Geometry: final body of the model. Coordinates: model frame, mm. Coordinates: 2 decimals unless noted, no trailing zeros. Write each loop counter-clockwise with the first axis right and the second up, starting at its lowest first coordinate (ties: lowest second). Pieces come first, ordered by that corner, then holes.
from build123d import *

# Parameters (mm, degrees)
F0_W     = 20
F0_H     = 20
F1_DEPTH = 20
F4_DEPTH = 15


with BuildPart() as f1:
    # F0 (on Top) → F1 (new body)
    with BuildSketch(Plane.XY):
        Rectangle(F0_W, F0_H)
    extrude(amount=F1_DEPTH)

    # F3 (on 3pt) → F4 (cut, symmetric)
    with BuildSketch(Plane(origin=(0, 0, 0), x_dir=(-0.7071067812, 0.7071067812, 0), z_dir=(0.7071067812, 0.7071067812, 0))):
        Polygon((14.1421356237, 0), (14.1421356237, 20), (0, 20), align=None)
    extrude(amount=F4_DEPTH, both=True, mode=Mode.SUBTRACT)


solid = f1.part
Item 1: Section B-B, the plane x = -3. Output: boundary loops of the cut face in (y, z), plus the area to 4 significant figures.
Derived:
outline: (-10, 0) - (10, 0) - (10, 7) - (-3, 20) - (-10, 20) - close
area: 315.5 mm2
Item 2: Pin query (flat end, axial travel): pin 1 (4 mm diameter, centred on x = -6, z = 5.5, fed in from +Y); pin 2 (12 mm diameter, centred on x = -6, z = 15, fed in from +Y). Return the tip coordinate at first contact, or that it passes through.
Derived:
pin 1: stops at y = 10
pin 2: stops at y = 7.49
Item 3: Section A-A, the plane z = 9.25. Output: boundary loops of the cut face in (x, y), plus the area to 3 significant figures.
Derived:
outline: (-10, -10) - (10, -10) - (10, 10) - (-0.75, 10) - (-10, 0.75) - close
area: 357 mm2
Item 4: Material intervals for probe 1 along Y at (x, z) = (-4.25, 16.75); probe 2 along X at (y, z) = (4.25, 10.5); probe 3 along Z at (x, y) = (-3, 8.25), sorted ascending.
Derived:
probe 1: y = -10 to -1
probe 2: x = -5.25 to 10
probe 3: z = 0 to 8.75
